from build123d import *

# Parameters (mm, degrees)
SKETCH1_W           = 100
SKETCH1_H           = 100
BOSS_EXTRUDE1_DEPTH = 1
SKETCH2_W           = 50
SKETCH2_H           = 20
CUT_EXTRUDE1_DEPTH  = 1
SKETCH3_R           = 5
SKETCH3_R_2         = 15
CUT_EXTRUDE2_DEPTH  = 1


with BuildPart() as part:
    # Sketch1 → Boss-Extrude1 (new body)
    with BuildSketch(Plane(origin=(0, 0, 0), x_dir=(1, 0, 0), z_dir=(0, 1, 0))):
        Rectangle(SKETCH1_W, SKETCH1_H)
    extrude(amount=BOSS_EXTRUDE1_DEPTH)

    # Sketch2 → Cut-Extrude1 (cut)
    with BuildSketch(Plane(origin=(0, 1, 0), x_dir=(1, 0, 0), z_dir=(0, 1, 0))):
        Rectangle(SKETCH2_W, SKETCH2_H)
    extrude(amount=-CUT_EXTRUDE1_DEPTH, mode=Mode.SUBTRACT)

    # Sketch3 → Cut-Extrude2 (cut)
    with BuildSketch(Plane(origin=(0, 1, 0), x_dir=(1, 0, 0), z_dir=(0, 1, 0))):
        with Locations(Location((0, 30, 0), (0, 0, 270))):
            Circle(SKETCH3_R)
        with Locations(Location((0, -30, 0), (0, 0, 270))):
            Circle(SKETCH3_R_2)
    extrude(amount=-CUT_EXTRUDE2_DEPTH, mode=Mode.SUBTRACT)


solid = part.part
Read the model definition and answer for the solid it produces. Units are mm, in the model's axes. Coordinates: 2 decimals unless noted, no trailing zeros. Loops run counter-clockwise (first coordinate to the right, second up) from the corner with the lowest first, then second, coordinate; pieces in that order, holes last.
Q1. The part is cut by section B-B on x = 0. Write down the section's boundary in (y, z).
Q2. The mould has two halves that part along X. Classify faces 1 (the face through (12.65, 0.51, 38.06)), 2 (the face through (-1, 0, -12)): +X half, -X half, draft (parallel to the pull), parting line (faces both ways), or undercut.
Q3. The part is cut by section D-D on z = -30. Write down the section's boundary in (x, y).
Q4. The part is cut by section A-A on z = 30. Write down the section's boundary in (x, y), and give its area (3 significant figures).
Q5. The part is cut by section C-C on y = 0.8. Write down the section's boundary in (x, z), and give its area (3 significant figures).
Q6. Consider probe 1 along X at (y, z) = (0.45, 30); probe 2 along Z at (x, y) = (-6.5, 0.65); probe 3 along X at (y, z) = (0.45, 8). Determine where each line is inside the solid, lowest interval first.
Results below:
1. outline: (0, -50) - (1, -50) - (1, -35) - (0, -35) - close; (0, -25) - (1, -25) - (1, -10) - (0, -10) - close; (0, 10) - (1, 10) - (1, 15) - (0, 15) - close; (0, 45) - (1, 45) - (1, 50) - (0, 50) - close
2. face 1: undercut
2. face 2: draft
3. outline: (-50, 0) - (-5, 0) - (-5, 1) - (-50, 1) - close; (5, 0) - (50, 0) - (50, 1) - (5, 1) - close
4. outline: (-50, 0) - (-15, 0) - (-15, 1) - (-50, 1) - close; (15, 0) - (50, 0) - (50, 1) - (15, 1) - close
4. area: 70.0 mm2
5. outline: (-50, -50) - (50, -50) - (50, 50) - (-50, 50) - close; hole (-25, -10) - (25, -10) - (25, 10) - (-25, 10) - close; hole circle Ø30 at (0, 30); hole circle Ø10 at (0, -30)
5. area: 8,210 mm2
6. probe 1: x = -50 to -15, 15 to 50
6. probe 2: z = -50 to -10, 10 to 16.48, 43.52 to 50
6. probe 3: x = -50 to -25, 25 to 50
